Read the model definition and answer for the solid it produces. Units are mm, in the model's axes. Face numbers are marked on the shaded views. A direction names the side the tool comes from. Coordinates: 2 decimals unless noted, no trailing zeros. Loops run counter-clockwise (first coordinate to the right, second up) from the corner with the lowest first, then second, coordinate; pieces in that order, holes last. Notation, with made-up numbers: (-25, 14) -> (11, 14) arc R32 cw to (11, 48) -> close; hole circle Ø6 at (84.25, -35.75). An arc over 180 degrees is marked (long way). Answer in a Markdown table with one row per item.
```python
from build123d import *

# Parameters (mm, degrees)
F_1_8_0_125_DIAMETER_HOLE1_D = 3.175
CIRPATTERN1_COUNT            = 8


with BuildPart() as part:
    # Sketch1 → Revolve1 (revolve)
    with BuildSketch(Plane.XY):
        Polygon((0, 38.1), (0, 19.05), (-127, 19.05), (-127, 38.1), (-123.825, 38.1), (-123.825, 22.225), (-3.175, 22.225), (-3.175, 38.1), align=None)
    revolve(axis=Axis((-152.49, 0, 0), (1, 0, 0)))

    # 1/8 (0.125) Diameter Hole1 (through all)
    with Locations(Plane(origin=(0, 0, 0), x_dir=(0, 0, -1), z_dir=(1, 0, 0))):
        with Locations((0, 31.75)):
            f_1_8_0_125_diameter_hole1 = Hole(F_1_8_0_125_DIAMETER_HOLE1_D / 2)

    # CirPattern1: 1/8 (0.125) Diameter Hole1 ×8 about axis
    cirpattern1_axis = Axis((0, 0, 0), (1, 0, 0))
    for i in range(1, CIRPATTERN1_COUNT):
        add(f_1_8_0_125_diameter_hole1.rotate(cirpattern1_axis, i * 360 / CIRPATTERN1_COUNT), mode=Mode.SUBTRACT)


solid = part.part
```
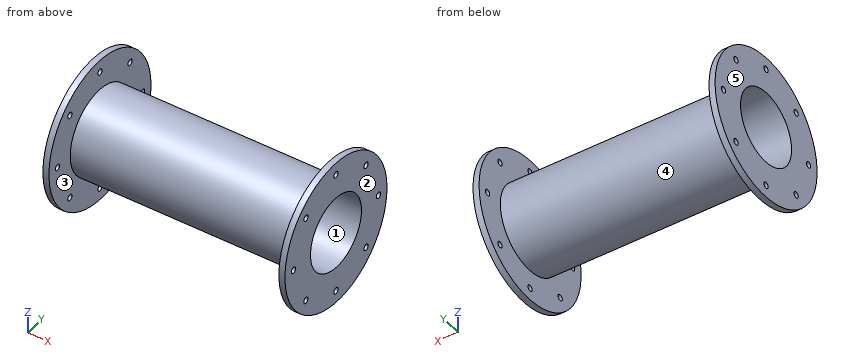
1. The mould has two halves that part along X. Classify the marked faces 1, 2 and 3: pulls with the +X half, pulls with the -X half, needs draft (parallel to the pull), parting line crosses it, or undercut.
A:
| item | result |
|---|---|
| face 1 | needs draft |
| face 2 | pulls with the +X half |
| face 3 | undercut |
2. A cutting plane is placed at C-C on z = -14. Give the vertices of the cut face in (x, y) (3 decimals), and give its area (3 significant figures).
A:
| item | result |
|---|---|
| outline | (-127, -35.435) -> (-123.825, -35.435) -> (-123.825, -17.261) -> (-3.175, -17.261) -> (-3.175, -35.435) -> (0, -35.435) -> (0, -12.919) -> (-127, -12.919) -> close; (-127, 12.919) -> (0, 12.919) -> (0, 35.435) -> (-3.175, 35.435) -> (-3.175, 17.261) -> (-123.825, 17.261) -> (-123.825, 35.435) -> (-127, 35.435) -> close |
| area | 1,330 mm2 |
3. A cutting plane is placed at D-D on x = -101.5. Give the vertices of the cut face in (y, z) (3 decimals), and give its area (3 significant figures).
A:
| item | result |
|---|---|
| outline | circle Ø44.45 at (0, 0); hole circle Ø38.1 at (0, 0) |
| area | 412 mm2 |
4. A cutting plane is placed at A-A on y = 0. Count the separate pieces of the cut face and the enclosed holes in it, and give its area (3 significant figures).
A:
| item | result |
|---|---|
| separate pieces | 6 |
| enclosed holes | 0 |
| area | 968 mm2 |
5. Given pin 1 Ø23 at (y, z) = (15.5, 13) entering from +X; pin 2 Ø4 at (x, y) = (-92, -17) entering from -Z; pin 3 Ø1 at (x, z) = (-14.5, 20.5) entering from -Y; pin 4 Ø1.5 at (x, z) = (-90.5, 12) entering from +Y, each flat-ended and moving along its own axis, determine where each tip first touches the part or whether it passes through.
A:
| item | result |
|---|---|
| pin 1 | stops at x = 0 |
| pin 2 | stops at z = -16.4 |
| pin 3 | stops at y = -9.69 |
| pin 4 | stops at y = 19.17 |
6. Find the intervals of material crossed by probe 1 along X at (y, z) = (32, 17) (3 decimals); probe 2 along Z at (x, y) = (-93, -8); probe 3 along Y at (x, z) = (-28, 11), in increasing order.
A:
| item | result |
|---|---|
| probe 1 | x = -127 to -123.825, -3.175 to 0 |
| probe 2 | z = -20.74 to -17.29, 17.29 to 20.74 |
| probe 3 | y = -19.31 to -15.55, 15.55 to 19.31 |
7. A tool of negligible diameter and unlimited length cuts with its end or side. For the marked faces 4 and 5, from which of +Z, -Z, +X, -X, +Y, -Y can it reach the whole face along a straight path? Write none if from no direction.
A:
| item | result |
|---|---|
| face 4 | none |
| face 5 | +Z, -Z, -X, +Y, -Y |
